from build123d import *

# Parameters (mm, degrees)
BOSS_EXTRUDE1_DEPTH     = 107
SKETCH2_R               = 2.5
CUT_EXTRUDE1_DEPTH      = 336.0337743
CUT_EXTRUDE4_REACH      = 337.034
SKETCH5_W               = 15.542799326
SKETCH5_H               = 10
SKETCH5_W_2             = 18.63674205
CUT_EXTRUDE5_DEPTH      = 255.70554643
CUT_EXTRUDE5_DEPTH_BACK = 255.70554643


with BuildPart() as part:
    # Sketch1 → Boss-Extrude1 (new body)
    with BuildSketch(Plane(origin=(0, 0, 0), x_dir=(1, 0, 0), z_dir=(0, 1, 0))):
        with BuildLine():
            Line((0, 0), (0, -8))
            Line((0, -8), (30, -8))
            ThreePointArc((30, -8), (149.5, -106.759683035), (269, -8))
            Line((269, -8), (299, -8))
            Line((299, -8), (299, 0))
            Line((299, 0), (269, 0))
            Line((269, 0), (269, 15))
            ThreePointArc((269, 15), (267.535533906, 18.535533906), (264, 20))
            Line((264, 20), (256.5, 20))
            ThreePointArc((256.5, 20), (149.5, -87.000008561), (42.5, 20))
            Line((42.5, 20), (35, 20))
            ThreePointArc((35, 20), (31.464466094, 18.535533906), (30, 15))
            Line((30, 15), (30, 0))
            Line((30, 0), (0, 0))
        make_face()
    extrude(amount=BOSS_EXTRUDE1_DEPTH)

    # Sketch2 → Cut-Extrude1 (cut, through all)
    with BuildSketch(Plane(origin=(0, 0, 0), x_dir=(-1, 0, 0), z_dir=(0, 0, -1))):
        with Locations((-286.5, 87)):
            Circle(SKETCH2_R)
        with Locations((-286.5, 20)):
            Circle(SKETCH2_R)
        with Locations((-12.5, 87)):
            Circle(SKETCH2_R)
        with Locations((-12.5, 20)):
            Circle(SKETCH2_R)
    extrude(amount=-CUT_EXTRUDE1_DEPTH, mode=Mode.SUBTRACT)

    # Cut-Extrude4: up to this face of the body (flat: up to its plane)
    cut_extrude4_end = Plane(part.part.faces().sort_by_distance((260.25, 53.5, -20))[0])
    # Sketch5 → Cut-Extrude4 (cut, up to the picked face)
    with BuildSketch(Plane(origin=(0, 0, 0), x_dir=(-1, 0, 0), z_dir=(0, 0, -1)), mode=Mode.PRIVATE) as cut_extrude4_sk1:
        with Locations((-261.228600337, 86.535453814)):
            Rectangle(SKETCH5_W, SKETCH5_H)
    cut_extrude4_tool1 = split(extrude(cut_extrude4_sk1.sketch, amount=CUT_EXTRUDE4_REACH, mode=Mode.PRIVATE), bisect_by=cut_extrude4_end, keep=Keep.BOTH, mode=Mode.PRIVATE)
    # Sketch5 → Cut-Extrude4 (cut, up to the picked face)
    with BuildSketch(Plane(origin=(0, 0, 0), x_dir=(-1, 0, 0), z_dir=(0, 0, -1)), mode=Mode.PRIVATE) as cut_extrude4_sk2:
        with Locations((-259.681628975, 19.008712967)):
            Rectangle(SKETCH5_W_2, SKETCH5_H)
    cut_extrude4_tool2 = split(extrude(cut_extrude4_sk2.sketch, amount=CUT_EXTRUDE4_REACH, mode=Mode.PRIVATE), bisect_by=cut_extrude4_end, keep=Keep.BOTH, mode=Mode.PRIVATE)
    # Sketch5 → Cut-Extrude4 (cut, up to the picked face)
    with BuildSketch(Plane(origin=(0, 0, 0), x_dir=(-1, 0, 0), z_dir=(0, 0, -1)), mode=Mode.PRIVATE) as cut_extrude4_sk3:
        with Locations((-39.318371025, 19.008712967)):
            Rectangle(SKETCH5_W_2, SKETCH5_H)
    cut_extrude4_tool3 = split(extrude(cut_extrude4_sk3.sketch, amount=CUT_EXTRUDE4_REACH, mode=Mode.PRIVATE), bisect_by=cut_extrude4_end, keep=Keep.BOTH, mode=Mode.PRIVATE)
    # Sketch5 → Cut-Extrude4 (cut, up to the picked face)
    with BuildSketch(Plane(origin=(0, 0, 0), x_dir=(-1, 0, 0), z_dir=(0, 0, -1)), mode=Mode.PRIVATE) as cut_extrude4_sk4:
        with Locations((-37.771399663, 86.535453814)):
            Rectangle(SKETCH5_W, SKETCH5_H)
    cut_extrude4_tool4 = split(extrude(cut_extrude4_sk4.sketch, amount=CUT_EXTRUDE4_REACH, mode=Mode.PRIVATE), bisect_by=cut_extrude4_end, keep=Keep.BOTH, mode=Mode.PRIVATE)
    add(cut_extrude4_tool1.solids().sort_by(Axis((261.2286, 86.535454, 0), (0, 0, -1)))[0], mode=Mode.SUBTRACT)
    add(cut_extrude4_tool2.solids().sort_by(Axis((259.681629, 19.008713, 0), (0, 0, -1)))[0], mode=Mode.SUBTRACT)
    add(cut_extrude4_tool3.solids().sort_by(Axis((39.318371, 19.008713, 0), (0, 0, -1)))[0], mode=Mode.SUBTRACT)
    add(cut_extrude4_tool4.solids().sort_by(Axis((37.7714, 86.535454, 0), (0, 0, -1)))[0], mode=Mode.SUBTRACT)

    # Sketch8 → Cut-Extrude5 (cut, two sides: drawn at the far end of the back side and taken through both)
    with BuildSketch(Plane(origin=(152.698962186, 0, 153.519285181), x_dir=(0.7089984938103423, 0, -0.7052099940972661), z_dir=(0.7052099940972661, 0, 0.7089984938103423)).offset(-CUT_EXTRUDE5_DEPTH_BACK)):
        with BuildLine():
            Line((138.078914882, 99.021927615), (178.078914882, 99.021927615))
            ThreePointArc((178.078914882, 99.021927615), (181.614448788, 97.557461521), (183.078914882, 94.021927615))
            Line((183.078914882, 94.021927615), (183.078914882, 16.437469362))
            ThreePointArc((183.078914882, 16.437469362), (181.614448788, 12.901935456), (178.078914882, 11.437469362))
            Line((178.078914882, 11.437469362), (138.078914882, 11.437469362))
            ThreePointArc((138.078914882, 11.437469362), (134.543380976, 12.901935456), (133.078914882, 16.437469362))
            Line((133.078914882, 16.437469362), (133.078914882, 94.021927615))
            ThreePointArc((133.078914882, 94.021927615), (134.543380976, 97.557461521), (138.078914882, 99.021927615))
        make_face()
    extrude(amount=CUT_EXTRUDE5_DEPTH + CUT_EXTRUDE5_DEPTH_BACK, mode=Mode.SUBTRACT)


solid = part.part
Geometry check sheet. Reference: the model listing, model coordinates, mm. A direction names the side the tool comes from. Round coordinates to 2 decimals unless told otherwise and drop trailing zeros. Loops run counter-clockwise (first coordinate to the right, second up) from the corner with the lowest first, then second, coordinate; pieces in that order, holes last. Notation, with made-up numbers: (10, -38) - (42, -38) arc R26 ccw to (42, -3) - close; hole circle Ø1 at (4, 48). An arc over 180 degrees is marked (long way). Answer as CSV lines item,"result".
(1) Depth check by flat-ended pin: pin 1 Ø1.5 at (x, y) = (187, 88) entering from -Z; pin 2 Ø4 at (x, y) = (225.5, 63.5) entering from -Z; pin 3 Ø8 at (y, z) = (37, 65.5) entering from -X; pin 4 Ø4.5 at (x, y) = (12.5, 87) entering from -Z. Enter the tip coordinate at first touch or a pass-through.
Output values:
pin 1,"stops at z = 79.93"
pin 2,"stops at z = 53.25"
pin 3,"stops at x = 54.81"
pin 4,"passes through"
(2) Cross-section at A-A, the plane y = 55. Enter the section's corners in (x, z).
Output values:
outline,"(0, 0) - (30, 0) - (30, -15) arc R5 ccw to (35, -20) - (42.5, -20) arc R107 cw to (233.6, 46.15) - (246.25, 58.87) arc R121.68 ccw to (30, 8) - (0, 8) - close; (255.15, -3.08) arc R107 cw to (256.5, -20) - (264, -20) arc R5 ccw to (269, -15) - (269, 0) - (299, 0) - (299, 8) - (269, 8) arc R121.68 ccw to (268.52, 10.36) - close"
(3) Cross-section at C-C, the plane y = 8.5. Enter the section's corners in (x, z).
Output values:
outline,"(0, 0) - (30, 0) - (30, -15) arc R5 ccw to (35, -20) - (42.5, -20) arc R107 cw to (256.5, -20) - (264, -20) arc R5 ccw to (269, -15) - (269, 0) - (299, 0) - (299, 8) - (269, 8) arc R121.68 ccw to (30, 8) - (0, 8) - close"
(4) Cross-section at B-B, the plane z = 70. Enter the section's corners in (x, y), and give its area (3 significant figures).
Output values:
outline,"(62.35, 0) - (91.63, 0) - (91.63, 107) - (62.35, 107) - close; (207.37, 0) - (236.65, 0) - (236.65, 107) - (207.37, 107) - close"
area,"6,260 mm²"
(5) Material ranges on line 1 along Y through (x, z) = (12.5, 4); line 2 along Y through (x, z) = (262, -13); line 3 along Y through (x, z) = (244, 36), recorded low to high.
Output values:
line 1,"y = 0 to 17.5, 22.5 to 84.5, 89.5 to 107"
line 2,"y = 0 to 14.01, 24.01 to 81.54, 91.54 to 107"
line 3,"y = 0 to 11.44, 99.02 to 107"
(6) Set-up check for faces 1 (the face through (256.172, 52.369, -11.634)), 2 (the face through (269, 99, -7)), 3 (the face through (37, 14.009, -10)): record each of +Z, -Z, +X, -X, +Y, -Y from which the full face is reachable in a straight line by a thin tool's end or side.
Output values:
face 1,"-Z, +Y, -Y"
face 2,"-Z, +X, +Y, -Y"
face 3,"-Z, +X, -X"
(7) Release check for a two-part mould opening along X. For faces 4 (the face through (251, 99.022, 29)), 5 (the face through (0, 53, 4)), 6 (the face through (262, 81.535, -10)), 7 (the face through (269, 7, -7)) record: released by +X, released by -X, zero draft, split by the parting line, or undercut.
Output values:
face 4,"undercut"
face 5,"released by -X"
face 6,"zero draft"
face 7,"released by +X"
(8) Cross-section at D-D, the plane x = 149.5. Enter the section's corners in (y, z).
Output values:
outline,"(0, 87) - (107, 87) - (107, 106.76) - (0, 106.76) - close"
